Here's how the part is built. I have some questions about the finished solid (model axes, mm). A direction names the side the tool comes from. Round coordinates to 2 decimals unless told otherwise and drop trailing zeros. Loops run counter-clockwise (first coordinate to the right, second up) from the corner with the lowest first, then second, coordinate; pieces in that order, holes last. Notation, with made-up numbers: M -38.5,28.25 L 19.5,28.25 A24 cw 19.5,67.25 Z; hole C 82.25,12.5 d9. An arc over 180 degrees is marked long. Answer as a JSON object with one key per item and string values.
from build123d import *

# Parameters (mm, degrees)
ESBO_O2_R                = 7.5
ESBO_O2_R_2              = 6.5
RESSALTO_EXTRUS_O1_DEPTH = 23.5
RESSALTO_EXTRUS_O2_DEPTH = 1


with BuildPart() as part:
    # Esboço2 → Ressalto-extrusão1 (new body)
    with BuildSketch(Plane.XY):
        Circle(ESBO_O2_R)
        Circle(ESBO_O2_R_2, mode=Mode.SUBTRACT)
    extrude(amount=RESSALTO_EXTRUS_O1_DEPTH)

    # Esboço3 → Ressalto-extrusão2 (add)
    with BuildSketch(Plane(origin=(-7.5, 0, 0), x_dir=(0, 0, -1), z_dir=(1, 0, 0))):
        with BuildLine():
            Line((5, 1.5), (0, 1.5))
            Line((0, 1.5), (0, 2.5))
            Line((0, 2.5), (5, 2.5))
            ThreePointArc((5, 2.5), (7.5, 0), (5, -2.5))
            Line((5, -2.5), (0, -2.5))
            Line((0, -2.5), (0, -1.5))
            Line((0, -1.5), (5, -1.5))
            ThreePointArc((5, -1.5), (6.5, 0), (5, 1.5))
        make_face()
        with BuildLine():
            Line((-28.5, 2.5), (-23.5, 2.5))
            Line((-23.5, 2.5), (-23.5, 1.5))
            Line((-23.5, 1.5), (-28.5, 1.5))
            ThreePointArc((-28.5, 1.5), (-30, 0), (-28.5, -1.5))
            Line((-28.5, -1.5), (-23.5, -1.5))
            Line((-23.5, -1.5), (-23.5, -2.5))
            Line((-23.5, -2.5), (-28.5, -2.5))
            ThreePointArc((-28.5, -2.5), (-31, 0), (-28.5, 2.5))
        make_face()
    extrude(amount=RESSALTO_EXTRUS_O2_DEPTH)


solid = part.part
Item 1: If we mould it in two halves opening along X, with no side actions, what happens to faces 1 (the face through (-7, 1.5, 26)), 2 (the face through (-5.158, -3.955, 11.586)), 3 (the face through (-7.5, 2, -4))? For each: pulls with the +X half, pulls with the -X half, needs draft (parallel to the pull), parting line crosses it, or undercut.
Resolved:
{"face 1": "needs draft", "face 2": "undercut", "face 3": "pulls with the -X half"}
Item 2: I want a section at D-D, the plane z = 11. Please give me the cut outline in (x, y), then the cut area to 3 significant figures.
Resolved:
{"outline": "C 0,0 d15; hole C 0,0 d13", "area": "44.0 mm²"}
Item 3: I want a section at C-C, the plane y = 0. Please give me the cut outline in (x, z).
Resolved:
{"outline": "M -7.5,-7.5 L -6.5,-7.5 L -6.5,-6.5 L -7.5,-6.5 Z; M -7.5,0 L -6.5,0 L -6.5,23.5 L -7.5,23.5 Z; M -7.5,30 L -6.5,30 L -6.5,31 L -7.5,31 Z; M 6.5,0 L 7.5,0 L 7.5,23.5 L 6.5,23.5 Z"}
Item 4: I want a section at A-A, the plane z = 25.5. Please give me the cut outline in (x, y).
Resolved:
{"outline": "M -7.5,-2.5 L -6.5,-2.5 L -6.5,-1.5 L -7.5,-1.5 Z; M -7.5,1.5 L -6.5,1.5 L -6.5,2.5 L -7.5,2.5 Z"}
Item 5: I want a section at B-B, the plane x = 0. Please give me the cut outline in (y, z).
Resolved:
{"outline": "M -7.5,0 L -6.5,0 L -6.5,23.5 L -7.5,23.5 Z; M 6.5,0 L 7.5,0 L 7.5,23.5 L 6.5,23.5 Z"}
Item 6: I'm going to push flat-ended pins straight in: pin 1 Ø0.8 at (x, z) = (-7, 27) entering from +Y; pin 2 Ø5.5 at (y, z) = (1, -4) entering from +X; pin 3 Ø5 at (x, y) = (2, 4.5) entering from +Z. Where does each tip first touch, or does it pass through?
Resolved:
{"pin 1": "y = 2.5", "pin 2": "x = -6.5", "pin 3": "z = 23.5"}
Item 7: Please list where these lines run through material, in increasing order: probe 1 along Y at (x, z) = (0, 8.25); probe 2 along Z at (x, y) = (-6.25, 2.5); probe 3 along X at (y, z) = (-3.75, 5.5). Write a range as from..to.
Resolved:
{"probe 1": "-7.5..-6.5, 6.5..7.5", "probe 2": "0..23.5", "probe 3": "-6.5..-5.31, 5.31..6.5"}
Item 8: On a 3-axis mill with a long thin cutter (end or side, diameter ignored), from which of +Z, -Z, +X, -X, +Y, -Y can I reach the whole of each face in a straight line? I mean faces 4 (the face through (-6.5, -2, 27)), 5 (the face through (-7, -2.5, -3)), 6 (the face through (-7, 0, 30)), 7 (the face through (-7, 2.5, -2)). Say none if no direction works.
Resolved:
{"face 4": "+Z, +X, +Y, -Y", "face 5": "-Z, +X, -X, -Y", "face 6": "+X, -X", "face 7": "-Z, +X, -X, +Y"}
